```python
from build123d import *

# Parameters (mm, degrees)
SKETCH1_R                   = 15.5067
BOSS_EXTRUDE1_DEPTH         = 2.9464
CUT_EXTRUDE1_REACH          = 24.127
CUT_EXTRUDE2_REACH          = 24.127
SKETCH3_W                   = 2.9591
SKETCH3_H                   = 7.9375
TAP_DRILL_FOR_4_HELICOIL1_D = 3.9878


with BuildPart() as part:
    # Sketch1 → Boss-Extrude1 (new body)
    with BuildSketch(Plane.XY):
        Circle(SKETCH1_R)
    extrude(amount=BOSS_EXTRUDE1_DEPTH)

    # Sketch2 → Cut-Extrude1 (cut, up to next)
    with BuildSketch(Plane.XY.offset(2.9464), mode=Mode.PRIVATE) as cut_extrude1_sk1:
        with BuildLine():
            Line((4.7625, 6.270444143), (4.7625, 4.783418626))
            ThreePointArc((4.7625, 4.783418626), (6.75, 0), (4.7625, -4.783418626))
            Line((4.7625, -4.783418626), (4.7625, -6.270444143))
            ThreePointArc((4.7625, -6.270444143), (0, -7.874), (-4.7625, -6.270444143))
            Line((-4.7625, -6.270444143), (-4.7625, -4.783418626))
            ThreePointArc((-4.7625, -4.783418626), (-6.75, 0), (-4.7625, 4.783418626))
            Line((-4.7625, 4.783418626), (-4.7625, 6.270444143))
            ThreePointArc((-4.7625, 6.270444143), (0, 7.874), (4.7625, 6.270444143))
        make_face()
    cut_extrude1_tool1 = extrude(cut_extrude1_sk1.sketch, amount=-CUT_EXTRUDE1_REACH, mode=Mode.PRIVATE) & part.part
    add(cut_extrude1_tool1.solids().sort_by_distance((0, 0, 2.9464))[0], mode=Mode.SUBTRACT)

    # Sketch3 → Cut-Extrude2 (cut, up to next)
    with BuildSketch(Plane(origin=(0, 0, 0), x_dir=(-1, 0, 0), z_dir=(0, 0, -1)), mode=Mode.PRIVATE) as cut_extrude2_sk1:
        with Locations((-9.41705, 0)):
            Rectangle(SKETCH3_W, SKETCH3_H)
    cut_extrude2_tool1 = extrude(cut_extrude2_sk1.sketch, amount=-CUT_EXTRUDE2_REACH, mode=Mode.PRIVATE) & part.part
    cut_extrude2 = cut_extrude2_tool1.solids().sort_by_distance((9.41705, 0, 0))[0]
    add(cut_extrude2, mode=Mode.SUBTRACT)

    # Mirror1: Cut-Extrude2 across plane
    add(cut_extrude2.mirror(Plane(origin=(0, 0, 0), x_dir=(0, 0, 1), z_dir=(1, 0, 0))), mode=Mode.SUBTRACT)

    # Tap Drill for #4 Helicoil1 (through all)
    with Locations(Plane.XY.offset(2.9464)):
        with Locations((0, 12.7), (0, -12.7)):
            Hole(TAP_DRILL_FOR_4_HELICOIL1_D / 2)


solid = part.part
```
Design review of the part built by this model. Coordinates are the model's own, in mm. A direction names the side the tool comes from. Give positions to 0.01 mm unless a question says otherwise; leave off trailing zeros. Loops run counter-clockwise (first coordinate to the right, second up) from the corner with the lowest first, then second, coordinate; pieces in that order, holes last. Notation, with made-up numbers: (39.5, 78.25) -> (48.5, 78.25) arc R19 cw to (48.5, 91.25) -> close; hole circle Ø7 at (-3, 13). An arc over 180 degrees is marked (long way). One line per item, written item: value.
Q1. Machinability: for faces 4 (the flat face through (7, -3, 0)), 5 (the flat face through (10.897, 0, 1)), which of the approach directions +Z, -Z, +X, -X, +Y, -Y give a long, thin tool a straight path to every point of the face, cutting with its end or side? Answer none if there is none.
Numbers:
face 4: -Z, +X, -X, +Y, -Y
face 5: +Z, -Z
Q2. We need section B-B on y = 0. Give the boundary of the cut face in (x, z).
Numbers:
outline: (-15.51, 0) -> (-10.9, 0) -> (-10.9, 2.95) -> (-15.51, 2.95) -> close; (-7.94, 0) -> (-6.75, 0) -> (-6.75, 2.95) -> (-7.94, 2.95) -> close; (6.75, 0) -> (7.94, 0) -> (7.94, 2.95) -> (6.75, 2.95) -> close; (10.9, 0) -> (15.51, 0) -> (15.51, 2.95) -> (10.9, 2.95) -> close
Q3. For pin 1 Ø1.5 at (x, z) = (9.5, 1.5) entering from +Y; pin 2 Ø1.6 at (y, z) = (5.5, 2) entering from +X; pin 3 Ø1.2 at (y, z) = (-5, 2) entering from -X, all flat-tipped, find the tip position at first contact; note any pin that passes through.
Numbers:
pin 1: stops at y = 12.8
pin 2: stops at x = 14.78
pin 3: stops at x = -14.87
Q4. We need section A-A on x = 0. Give the boundary of the cut face in (y, z).
Numbers:
outline: (-15.51, 0) -> (-14.69, 0) -> (-14.69, 2.95) -> (-15.51, 2.95) -> close; (-10.71, 0) -> (-7.87, 0) -> (-7.87, 2.95) -> (-10.71, 2.95) -> close; (7.87, 0) -> (10.71, 0) -> (10.71, 2.95) -> (7.87, 2.95) -> close; (14.69, 0) -> (15.51, 0) -> (15.51, 2.95) -> (14.69, 2.95) -> close
Q5. We need section D-D on x = 5.5. Give the boundary of the cut face in (y, z), and give its area (3 significant figures).
Numbers:
outline: (-14.5, 0) -> (-3.91, 0) -> (-3.91, 2.95) -> (-14.5, 2.95) -> close; (3.91, 0) -> (14.5, 0) -> (14.5, 2.95) -> (3.91, 2.95) -> close
area: 62.4 mm^2
Q6. Draft analysis for pull direction X (two halves, no side actions). For faces 1 (the cylindrical face through (-3.36, -15.14, 1.45)), 2 (the flat face through (7, -3, 2.946)), 3 (the flat face through (9, -3.969, 1)), state which applies: pulls with the +X half, pulls with the -X half, needs draft (parallel to the pull), parting line crosses it, or undercut.
Numbers:
face 1: parting line crosses it
face 2: needs draft
face 3: undercut
Q7. We need section C-C on z = 1.3. Give the boundary of the cut face in (x, y).
Numbers:
outline: circle Ø31.01 at (0, 0); hole (-10.9, -3.97) -> (-7.94, -3.97) -> (-7.94, 3.97) -> (-10.9, 3.97) -> close; hole (-4.76, -6.27) arc R7.87 ccw to (4.76, -6.27) -> (4.76, -4.78) arc R6.75 ccw to (4.76, 4.78) -> (4.76, 6.27) arc R7.87 ccw to (-4.76, 6.27) -> (-4.76, 4.78) arc R6.75 ccw to (-4.76, -4.78) -> close; hole circle Ø3.99 at (0, -12.7); hole circle Ø3.99 at (0, 12.7); hole (7.94, -3.97) -> (10.9, -3.97) -> (10.9, 3.97) -> (7.94, 3.97) -> close
Q8. For L1, parallel to Y at x = 0, z = 2.35; L2, parallel to X at y = -0.5, z = 2.3; L3, parallel to X at y = 13, z = 2.45, list the stretches that pass through material, from the lowest coordinate up.
Numbers:
L1: y = -15.51 to -14.69, -10.71 to -7.87, 7.87 to 10.71, 14.69 to 15.51
L2: x = -15.5 to -10.9, -7.94 to -6.73, 6.73 to 7.94, 10.9 to 15.5
L3: x = -8.45 to -1.97, 1.97 to 8.45
